Autodesk Inventor part; units mm, degrees
ref_plane "YZ Plane" through (0, 0, 0) normal (1, 0, 0) x (0, 1, 0)
ref_plane "XZ Plane" through (0, 0, 0) normal (0, 1, 0) x (-1, 0, 0)
ref_plane "XY Plane" through (0, 0, 0) normal (0, 0, 1) x (1, 0, 0)
sketch "Sketch1" plane through (0, 0, 0) normal (0, 0, 1) x (1, 0, 0)
  line L0 (-75, -6) -> (75, -6)
  line L1 (75, -6) -> (75, 6)
  line L2 (75, 6) -> (-75, 6)
  line L3 (-75, 6) -> (-75, -6)
  line L4 (-75, -6) -> (75, 6) construction
  line L5 (75, -6) -> (-75, 6) construction
  point P0 (0, 0)
  dimension "d0" = 150
  dimension "d1" = 12
extrude "Extrusion1" add sketch "Sketch1" along normal blind 1
sketch "Sketch2" plane through (0, 0, 1) normal (0, 0, 1) x (1, 0, 0)
  line L0 (-66.5, 0) -> (-53.5, 0) construction
  line L1 (-53.5, 0) -> (53.5, 0) construction
  line L2 (53.5, 0) -> (66.5, 0) construction
  point P0 (0, 0)
  point P1 (0, 0)
  dimension "d4" = 133
  dimension "d5" = 13
  dimension "d6" = 13
hole "Hole1" at (-66.5, 0, 1) at (-53.5, 0, 1) at (66.5, 0, 1) at (53.5, 0, 1) direction (0, 0, -1) diameter 3.4 depth 8 tip angle 118
sketch "Sketch4" plane through (0, 0, 1) normal (0, 0, 1) x (1, 0, 0)
  line L0 (-37.5, 0) -> (37.5, 0) construction
  point P0 (0, 0)
  point P1 (0, 0)
  dimension "d21" = 75
hole "Hole3" at (-37.5, 0, 1) at (37.5, 0, 1) direction (0, 0, -1) diameter 4.5 depth 8 tip angle 118
sketch "Sketch6" plane through (-75, -6, 0) normal (-1, 0, 0) x (0, 0, 1)
  line L0 (1, 0) -> (1, 12)
  line L1 (0, 0) -> (1, 0)
  line L2 (1, 0) -> (1, 12)
  line L3 (1, 12) -> (0, 12)
  line L4 (0, 12) -> (0, 0)
  point P0 (0, 6)
extrude "Extrusion2" add sketch "Sketch6" along normal blind 20
sketch "Sketch7" plane through (0, 0, 1) normal (0, 0, 1) x (1, 0, 0)
  line L0 (-95, -6) -> (-95, 6)
  point P0 (0, 0)
  point P1 (-85, 0)
  dimension "d39" = 10
hole "Hole5" at (-85, 0, 1) direction (0, 0, -1) diameter 5.5 depth 8 tip angle 118
properties part number "CU6" material "Copper"
Can you work these out from the model? Positions are in its coordinate system, mm. Give positions to 0.01 mm unless a question says otherwise; leave off trailing zeros. Order: outer loops, then holes, each group sorted by start corner. A loop starts at its lowest first (then second) coordinate and runs counter-clockwise, first axis right, second up. Notation, with made-up numbers: (60, 62.25) - (111, 62.25) arc R13 ccw to (111, 82.25) - close; hole circle Ø3 at (72.25, 47.25). An arc over 180 degrees is marked (long way). Use a Markdown table: item, result. Add a question column.
Q1. If we mould it in two halves opening along X, with no side actions, what happens to faces 1 (the flat face through (-9, 0, 1)), 2 (the cylindrical face through (-82.315, 0.596, 0.493))? For each: released by +X, released by -X, zero draft, split by the parting line, or undercut.
Q2. If we section it at A-A on x = -37.5: Write out the boundary of the cut face in (y, z).
Q3. If we section it at C-C on z = 0.55: Write out the boundary of the cut face in (x, y).
Q4. Please list where these lines run through material, in increasing order: line 1 along Y through (x, z) = (37.5, 0.75); line 2 along Y through (x, z) = (52.5, 0.05).
Q5. If we section it at D-D on x = 66.5: Write out the boundary of the cut face in (y, z), plus the area to 3 significant figures.
Q6. If we section it at B-B on y = 0: Count the separate pieces of the cut face and the enclosed holes in it, plus the area to 3 significant figures.
Answers follow:
| question | item | result |
|---|---|---|
| 1 | face 1 | zero draft |
| 1 | face 2 | undercut |
| 2 | outline | (-6, 0) - (-2.25, 0) - (-2.25, 1) - (-6, 1) - close; (2.25, 0) - (6, 0) - (6, 1) - (2.25, 1) - close |
| 3 | outline | (-95, -6) - (75, -6) - (75, 6) - (-95, 6) - close; hole circle Ø5.5 at (-85, 0); hole circle Ø3.4 at (-66.5, 0); hole circle Ø3.4 at (-53.5, 0); hole circle Ø4.5 at (-37.5, 0); hole circle Ø4.5 at (37.5, 0); hole circle Ø3.4 at (53.5, 0); hole circle Ø3.4 at (66.5, 0) |
| 4 | line 1 | y = -6 to -2.25, 2.25 to 6 |
| 4 | line 2 | y = -6 to -1.37, 1.37 to 6 |
| 5 | outline | (-6, 0) - (-1.7, 0) - (-1.7, 1) - (-6, 1) - close; (1.7, 0) - (6, 0) - (6, 1) - (1.7, 1) - close |
| 5 | area | 8.60 mm^2 |
| 6 | separate pieces | 8 |
| 6 | enclosed holes | 0 |
| 6 | area | 142 mm^2 |
